Could you check a few things on this drawing? It's one solid part, dimensions in mm from its lowest x, y, z. Give positions to 0.01 mm unless a question says otherwise; leave off trailing zeros. Loops run counter-clockwise (first coordinate to the right, second up) from the corner with the lowest first, then second, coordinate; pieces in that order, holes last. Notation, with made-up numbers: (-38, 87.25) - (-31, 87.25) arc R18 ccw to (-31, 101.25) - close; hole circle Ø8 at (-12.75, 7.5). An arc over 180 degrees is marked (long way). One line per item, written item: value. Start each with the question number.
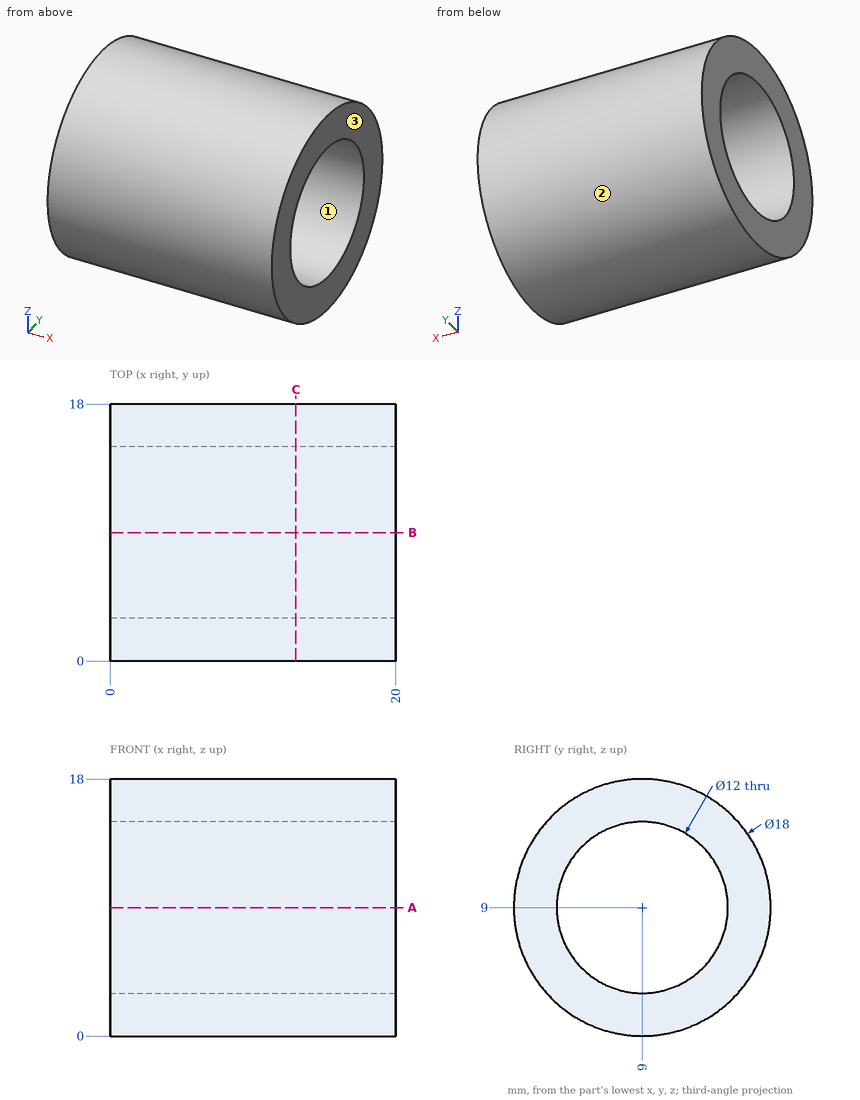
(1) Please list where these lines run through material, in increasing order: probe 1 along Y at (x, z) = (4.25, 9); probe 2 along Z at (x, y) = (9, 10.25); probe 3 along Z at (x, y) = (9.75, 7). Write a range as from..to.
(2) Will these pins go through, and if not, where does the flat tip stop? pin 1 (4 mm diameter, centred on x = 14, z = 14.5, fed in from +Y); pin 2 (10 mm diameter, centred on x = 15.5, y = 16, fed in from -Z); pin 3 (1 mm diameter, centred on x = 17.5, y = 3.5, fed in from +Z); pin 4 (9.5 mm diameter, centred on y = 9, z = 9, fed in from -X).
(3) If we section it at A-A on z = 9: List the corners of the cut face in (x, y) for me, plus the area to 3 significant figures.
(4) If we section it at C-C on x = 13: List the corners of the cut face in (y, z) for me.
(5) If we mould it in two halves opening along Z, with no side actions, what happens to the marked faces 1, 2 and 3? For each: pulls with the +Z half, pulls with the -Z half, needs draft (parallel to the pull), parting line crosses it, or undercut.
Found:
1. probe 1: 0..3, 15..18
1. probe 2: 0.09..3.13, 14.87..17.91
1. probe 3: 0.23..3.34, 14.66..17.77
2. pin 1: y = 17.29
2. pin 2: z = 0.23
2. pin 3: z = 16.48
2. pin 4: through
3. outline: (0, 0) - (20, 0) - (20, 3) - (0, 3) - close; (0, 15) - (20, 15) - (20, 18) - (0, 18) - close
3. area: 120 mm^2
4. outline: circle Ø18 at (9, 9); hole circle Ø12 at (9, 9)
5. face 1: undercut
5. face 2: parting line crosses it
5. face 3: needs draft
